Design review of the part built by this model. Coordinates are the model's own, in mm. Face numbers are marked on the shaded views. A direction names the side the tool comes from. Give positions to 0.01 mm unless a question says otherwise; leave off trailing zeros. Loops run counter-clockwise (first coordinate to the right, second up) from the corner with the lowest first, then second, coordinate; pieces in that order, holes last. Notation, with made-up numbers: (52.5, 83.25) -> (100.5, 83.25) arc R26 ccw to (100.5, 108.25) -> close; hole circle Ø6 at (26, -4.5). An arc over 180 degrees is marked (long way). Use a Markdown table: item, result. Add a question column.
1. Add section C-C (y = 0). State the section outline as (x, z) points, and give its area (3 significant figures).
2. Add section D-D (x = -13.5). State the section outline as (y, z) points.
3. Draft analysis for pull direction X (two halves, no side actions). For the marked faces 4, 5, 6 and 7, state which applies: pulls with the +X half, pulls with the -X half, needs draft (parallel to the pull), parting line crosses it, or undercut.
4. For pin 1 Ø1.4 at (x, y) = (13.5, 0) entering from +Z; pin 2 Ø0.9 at (x, z) = (16.75, 3.875) entering from +Y; pin 3 Ø1.5 at (y, z) = (3.5, 6) entering from -X; pin 4 Ø1.2 at (x, z) = (-16.75, 3.875) entering from -Y, all flat-tipped, find the tip position at first contact; note any pin that passes through.
5. To check wall thickness, follow line 1 (X direction, y = 5.25, z = 3.75); line 2 (Z direction, x = 16.75, y = -5.9) (3 decimals); line 3 (X direction, y = -0.5, z = 0.5). State the ranges of each line that lie inside material, in increasing order.
6. For the marked faces 1, 2 and 3, list the 3-axis set-ups (+Z, -Z, +X, -X, +Y, -Y) from which the entire face can be reached by the end or side of a thin tool; tool diameter is ignored.
7. Add section B-B (z = 1.5). State the section outline as (x, y) points, and give its area (3 significant figures).
8. Add section A-A (y = 5). State the section outline as (x, z) points, and give its area (4 significant figures).
```python
from build123d import *

# Parameters (mm, degrees)
BOSS_EXTRUDE1_DEPTH = 7.75
SKETCH2_R           = 0.75
CUT_EXTRUDE1_DEPTH  = 22.43157717
BOSS_EXTRUDE2_DEPTH = 7.75
SKETCH4_R           = 0.75
CUT_EXTRUDE2_DEPTH  = 2
FILLET1_R           = 10
FILLET2_R           = 4
FILLET3_R           = 0.3


with BuildPart() as part:
    # Sketch1 → Boss-Extrude1 (new body)
    with BuildSketch(Plane.XY):
        Polygon((11.5, -6.5), (17, -6.5), (17, 10.5), (-17, 10.5), (-17, -6.5), (-11.5, -6.5), (-11.5, 6.5), (11.5, 6.5), align=None)
    extrude(amount=BOSS_EXTRUDE1_DEPTH)

    # Sketch2 → Cut-Extrude1 (cut, through all)
    with BuildSketch(Plane.XY.offset(7.75)):
        with Locations((-13.5, 0)):
            Circle(SKETCH2_R)
        with Locations(Location((13.5, 0, 0), (0, 0, 180))):
            Circle(SKETCH2_R)
    extrude(amount=-CUT_EXTRUDE1_DEPTH, mode=Mode.SUBTRACT)

    # Sketch3 → Boss-Extrude2 (add)
    with BuildSketch(Plane.XY):
        Polygon((-17, -1.5), (-22, -6.5), (-17, -6.5), align=None)
        Polygon((17, -1.5), (22, -6.5), (17, -6.5), align=None)
    extrude(amount=BOSS_EXTRUDE2_DEPTH)

    # Sketch4 → Cut-Extrude2 (cut)
    with BuildSketch(Plane.XZ.offset(6.5)):
        with Locations((-16.75, 3.875)):
            Circle(SKETCH4_R)
        with Locations(Location((16.75, 3.875, 0), (0, 0, 180))):
            Circle(SKETCH4_R)
    extrude(amount=-CUT_EXTRUDE2_DEPTH, mode=Mode.SUBTRACT)

    # Fillet1
    fillet1_edges = [part.edges().sort_by_distance(p)[0] for p in [
        (-17, -1.5, 3.875),
        (17, -1.5, 3.875),
    ]]
    fillet(fillet1_edges, radius=FILLET1_R)

    # Fillet2
    fillet2_edges = [part.edges().sort_by_distance(p)[0] for p in [
        (-17, 10.5, 3.875),
        (17, 10.5, 3.875),
    ]]
    fillet(fillet2_edges, radius=FILLET2_R)

    # Fillet3
    fillet3_edges = [part.edges().sort_by_distance(p)[0] for p in [
        (-22, -6.5, 3.875),
        (22, -6.5, 3.875),
    ]]
    fillet(fillet3_edges, radius=FILLET3_R)


solid = part.part
```
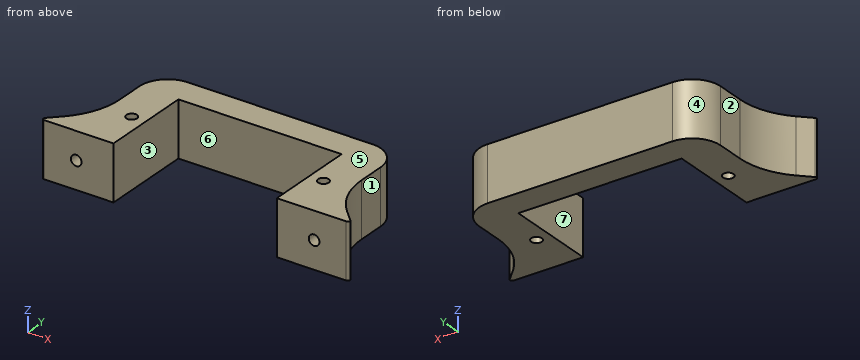
Taken from the geometry:
| question | item | result |
|---|---|---|
| 1 | outline | (-17.36, 0) -> (-14.25, 0) -> (-14.25, 7.75) -> (-17.36, 7.75) -> close; (-12.75, 0) -> (-11.5, 0) -> (-11.5, 7.75) -> (-12.75, 7.75) -> close; (11.5, 0) -> (12.75, 0) -> (12.75, 7.75) -> (11.5, 7.75) -> close; (14.25, 0) -> (17.36, 0) -> (17.36, 7.75) -> (14.25, 7.75) -> close |
| 1 | area | 67.5 mm^2 |
| 2 | outline | (-6.5, 0) -> (-0.75, 0) -> (-0.75, 7.75) -> (-6.5, 7.75) -> close; (0.75, 0) -> (10.47, 0) -> (10.47, 7.75) -> (0.75, 7.75) -> close |
| 3 | face 4 | pulls with the -X half |
| 3 | face 5 | needs draft |
| 3 | face 6 | undercut |
| 3 | face 7 | undercut |
| 4 | pin 1 | passes through |
| 4 | pin 2 | stops at y = 8.76 |
| 4 | pin 3 | stops at x = -17 |
| 4 | pin 4 | stops at y = -4.5 |
| 5 | line 1 | x = -17 to -11.5, 11.5 to 17 |
| 5 | line 2 | z = 0 to 3.125, 4.625 to 7.75 |
| 5 | line 3 | x = -17.51 to -14.06, -12.94 to -11.5, 11.5 to 12.94, 14.06 to 17.51 |
| 6 | face 1 | +Z, -Z, +X, +Y |
| 6 | face 2 | +Z, -Z, -X, +Y |
| 6 | face 3 | +Z, -Z, -Y |
| 7 | outline | (-21.49, -5.99) arc R0.3 ccw to (-21.28, -6.5) -> (-11.5, -6.5) -> (-11.5, 6.5) -> (11.5, 6.5) -> (11.5, -6.5) -> (21.28, -6.5) arc R0.3 ccw to (21.49, -5.99) -> (19.93, -4.43) arc R10 cw to (17, 2.64) -> (17, 6.5) arc R4 ccw to (13, 10.5) -> (-13, 10.5) arc R4 ccw to (-17, 6.5) -> (-17, 2.64) arc R10 cw to (-19.93, -4.43) -> close; hole circle Ø1.5 at (-13.5, 0); hole circle Ø1.5 at (13.5, 0) |
| 7 | area | 298 mm^2 |
| 8 | outline | (-17, 0) -> (-11.5, 0) -> (-11.5, 7.75) -> (-17, 7.75) -> close; (11.5, 0) -> (17, 0) -> (17, 7.75) -> (11.5, 7.75) -> close |
| 8 | area | 85.25 mm^2 |
